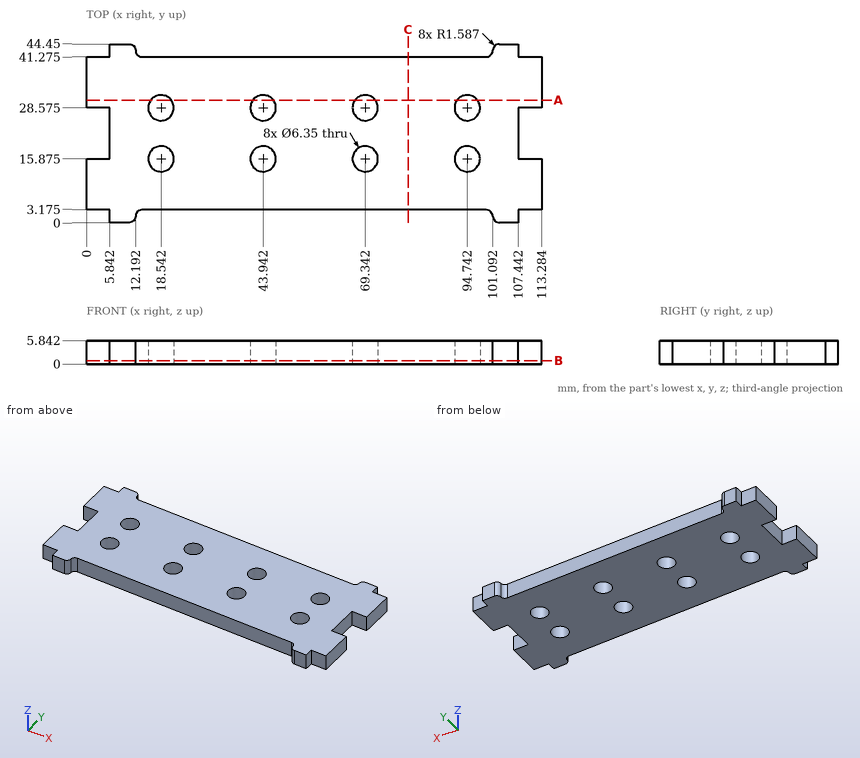
Check sheet for the drawn part. Datum: minimum x, y, z corner. Units: mm. Round coordinates to 2 decimals unless told otherwise and drop trailing zeros. Order: outer loops, then holes, each group sorted by start corner. A loop starts at its lowest first (then second) coordinate and runs counter-clockwise, first axis right, second up.
(1) Cross-section at A-A, the plane y = 30.5. Enter the section's corners in (x, z) (1 decimal), and give its area (3 significant figures).
(2) Cross-section at B-B, the plane z = 0.9. State how many separate pieces and enclosed holes the cut face has.
(3) Go/stop test with flat-tipped pins: P1, Ø1.8, axis at y = 21, z = 2, coming from the -X side; P2, Ø1.8, axis at x = 77, z = 2, coming from the +Y side (1 decimal); P3, Ø5.5, axis at x = 69.342, y = 15.875, coming from the -Z side. Record where each tip stops, or that it passes through.
(4) Cross-section at C-C, the plane x = 80. Enter the section's corners in (y, z) (1 decimal).
(5) Scan lines: probe 1 along X at (y, z) = (16.5, 2) (1 decimal); probe 2 along X at (y, z) = (29, 1) (1 decimal); probe 3 along Y at (x, z) = (27.5, 1.1) (1 decimal). Record each from-to range of solid material in increasing order.
Check sheet entries:
1. outline: (0, 0) - (16, 0) - (16, 5.8) - (0, 5.8) - close; (21.1, 0) - (41.4, 0) - (41.4, 5.8) - (21.1, 5.8) - close; (46.5, 0) - (66.8, 0) - (66.8, 5.8) - (46.5, 5.8) - close; (71.9, 0) - (92.2, 0) - (92.2, 5.8) - (71.9, 5.8) - close; (97.3, 0) - (113.3, 0) - (113.3, 5.8) - (97.3, 5.8) - close
1. area: 544 mm2
2. separate pieces: 1
2. enclosed holes: 8
3. P1: stops at x = 5.84
3. P2: stops at y = 41.3
3. P3: passes through
4. outline: (3.2, 0) - (41.3, 0) - (41.3, 5.8) - (3.2, 5.8) - close
5. probe 1: x = 5.8 to 15.4, 21.7 to 40.8, 47.1 to 66.2, 72.5 to 91.6, 97.9 to 107.4
5. probe 2: x = 0 to 15.4, 21.7 to 40.8, 47.1 to 66.2, 72.5 to 91.6, 97.9 to 113.3
5. probe 3: y = 3.2 to 41.3
